```python
from build123d import *

# Parameters (mm, degrees)
SKETCH1_W                 = 112.141
SKETCH1_H                 = 139.7
EXTRUDE1_DEPTH            = 6.35
SKETCH2_W                 = 44.45
SKETCH2_H                 = 19.05
SKETCH2_W_2               = 61.341
SKETCH2_H_2               = 127
SKETCH2_H_3               = 76.2
CUT_EXTRUDE1_DEPTH        = 6.35
FILLET1_R                 = 6.35
SKETCH5_W                 = 6.35
SKETCH5_H                 = 6.35
EXTRUDE2_DEPTH            = 6.35
FILLET2_R                 = 3.175
F_6_CLEARANCE_HOLE1_D     = 3.7973
F_6_CLEARANCE_HOLE1_DEPTH = 12.7
F_6_CLEARANCE_HOLE1_TIP   = 1.140824014
F_2_CLEARANCE_HOLE1_D     = 2.4384


with BuildPart() as part:
    # Sketch1 → Extrude1 (new body)
    with BuildSketch(Plane(origin=(0, 0, 0), x_dir=(1, 0, 0), z_dir=(0, 1, 0))):
        Rectangle(SKETCH1_W, SKETCH1_H)
    extrude(amount=EXTRUDE1_DEPTH)

    # Sketch2 → Cut-Extrude1 (cut)
    with BuildSketch(Plane(origin=(0, 6.35, 0), x_dir=(-1, 0, 0), z_dir=(0, 1, 0))):
        with Locations((33.8455, -60.325)):
            Rectangle(SKETCH2_W, SKETCH2_H)
        with Locations((33.8455, 60.325)):
            Rectangle(SKETCH2_W, SKETCH2_H)
        with Locations((-25.4, 0)):
            Rectangle(SKETCH2_W_2, SKETCH2_H_2)
        with Locations((33.8455, 0)):
            Rectangle(SKETCH2_W, SKETCH2_H_3)
    extrude(amount=-CUT_EXTRUDE1_DEPTH, mode=Mode.SUBTRACT)

    # Fillet1
    fillet1_edges = [part.edges().sort_by_distance(p)[0] for p in [
        (-11.6205, 3.175, -50.8),
        (-11.6205, 3.175, 50.8),
        (-5.2705, 3.175, 63.5),
        (-5.2705, 3.175, -63.5),
        (-11.6205, 3.175, -38.1),
        (-11.6205, 3.175, 38.1),
    ]]
    fillet(fillet1_edges, radius=FILLET1_R)

    # Sketch5 → Extrude2 (add)
    with BuildSketch(Plane.ZY.offset(56.0705)):
        with Locations((44.45, 3.175)):
            Rectangle(SKETCH5_W, SKETCH5_H)
        with Locations((-44.45, 3.175)):
            Rectangle(SKETCH5_W, SKETCH5_H)
    extrude(amount=EXTRUDE2_DEPTH)

    # Fillet2
    fillet2_edges = [part.edges().sort_by_distance(p)[0] for p in [
        (-62.4205, 6.35, 44.45),
        (-62.4205, 6.35, -44.45),
    ]]
    fillet(fillet2_edges, radius=FILLET2_R)

    # #6 Clearance Hole1
    with Locations(Plane(origin=(49.7205, 0, 66.675), x_dir=(0, 0, -1), z_dir=(0, -1, 0))):
        with Locations((0, 0), (133.35, 0)):
            Hole(F_6_CLEARANCE_HOLE1_D / 2, depth=F_6_CLEARANCE_HOLE1_DEPTH)
            with Locations((0, 0, -(F_6_CLEARANCE_HOLE1_DEPTH + F_6_CLEARANCE_HOLE1_TIP / 2))):  # 118° drill point
                Cone(0, F_6_CLEARANCE_HOLE1_D / 2, F_6_CLEARANCE_HOLE1_TIP, mode=Mode.SUBTRACT)

    # #2 Clearance Hole1 (through all)
    with Locations(Plane(origin=(-59.2455, 3.175, 47.625), x_dir=(1, 0, 0), z_dir=(0, 0, 1))):
        with Locations((0, 0)):
            Hole(F_2_CLEARANCE_HOLE1_D / 2)


solid = part.part
```
CAD build for the part. Positions are in the model's coordinates, mm. A direction names the side the tool comes from. Coordinates: 2 decimals unless noted, no trailing zeros. Order: outer loops, then holes, each group sorted by start corner. A loop starts at its lowest first (then second) coordinate and runs counter-clockwise, first axis right, second up. Notation, with made-up numbers: (41.5, 88.25) - (63.5, 88.25) arc R20 cw to (63.5, 100.25) - close; hole circle Ø1 at (12, 72). An arc over 180 degrees is marked (long way). Answer in a Markdown table with one row per item.
1. Drill centre lines: L1, parallel to Z at x = -32, y = 5; L2, parallel to Z at x = 3, y = 6; L3, parallel to Z at x = 49, y = 4. Where is each one in solid material? Low to high. Write a range as from..to.
Answer:
| item | result |
|---|---|
| L1 | -50.8..-38.1, 38.1..50.8 |
| L2 | -69.85..-63.5, 63.5..69.85 |
| L3 | -69.85..-68.43, -64.92..-63.5, 63.5..64.92, 68.43..69.85 |
2. Slice it at D-D, the plane x = -38. List the corners of the cut face in (y, z), then the cut area to 3 significant figures.
Answer:
| item | result |
|---|---|
| outline | (0, -50.8) - (6.35, -50.8) - (6.35, -38.1) - (0, -38.1) - close; (0, 38.1) - (6.35, 38.1) - (6.35, 50.8) - (0, 50.8) - close |
| area | 161 mm² |
3. 3-axis set-ups, long thin cutter, end or side, ignore diameter. For faces 5 (the face through (-37, 3, 38.1)), 6 (the face through (29, 3, 63.5)), 7 (the face through (-11.62, 3, 63)): which of +Z, -Z, +X, -X, +Y, -Y reach the whole face in a straight line?
Answer:
| item | result |
|---|---|
| face 5 | -X, +Y, -Y |
| face 6 | +X, +Y, -Y |
| face 7 | +Z, -X, +Y, -Y |
4. Flat gauge pins, fed straight in: P1, Ø1.5, axis at y = 4.5, z = 55.5, coming from the +X side; P2, Ø1, axis at y = 4, z = 36, coming from the -X side; P3, Ø3, axis at x = -41.5, y = 5, coming from the +Z side. Where does each tip first touch, or does it go through?
Answer:
| item | result |
|---|---|
| P1 | x = -5.27 |
| P2 | x = -13.76 |
| P3 | z = 50.8 |
5. Slice it at A-A, the plane x = 11. List the corners of the cut face in (y, z), then the cut area to 3 significant figures.
Answer:
| item | result |
|---|---|
| outline | (0, -69.85) - (6.35, -69.85) - (6.35, -63.5) - (0, -63.5) - close; (0, 63.5) - (6.35, 63.5) - (6.35, 69.85) - (0, 69.85) - close |
| area | 80.6 mm² |
6. Pull direction Z, two halves, no side cores. Call faces 1 (the face through (22, 3, -69.85)), 2 (the face through (-13.53, 3.13, 36.29)), 3 (the face through (-57.8, 3.1, 47.625)), 4 (the face through (-56.07, 3, 49)): +Z half, -Z half, draft (parallel to the pull), parting line (faces both ways), or undercut.
Answer:
| item | result |
|---|---|
| face 1 | -Z half |
| face 2 | undercut |
| face 3 | +Z half |
| face 4 | draft |
7. Slice it at C-C, the plane y = 1. Give the number of separate pieces and of enclosed holes in the cut face, then the cut area to 3 significant figures.
Answer:
| item | result |
|---|---|
| separate pieces | 1 |
| enclosed holes | 2 |
| area | 2,910 mm² |
